For this review, take the finished solid that the model builds, in its own axes (mm). Coordinates: 2 decimals unless noted, no trailing zeros. Loops run counter-clockwise (first coordinate to the right, second up) from the corner with the lowest first, then second, coordinate; pieces in that order, holes last. Notation, with made-up numbers: (-11.75, 77.5) - (44.25, 77.5) arc R17 ccw to (44.25, 93.5) - close; hole circle Ø11 at (36, 69). An arc over 180 degrees is marked (long way). Use one line per item in the form item = value. Start each with the question number.
1. To check wall thickness, follow probe 1 along X at (y, z) = (4, 0); probe 2 along Z at (x, y) = (-102, 1.35); probe 3 along X at (y, z) = (4, 7.5). State the ranges of each line that lie inside material, in increasing order.
2. Add section A-A on z = 20. Give the boundary of the cut face in (x, y), and give its area (3 significant figures).
3. Add section B-B on x = 33. Give the boundary of the cut face in (y, z), and give its area (3 significant figures).
4. Add section C-C on y = 3.65. Give the boundary of the cut face in (x, z) (3 decimals).
```python
from build123d import *

# Parameters (mm, degrees)
SKETCH1_W           = 266.7
SKETCH1_H           = 266.7
SKETCH1_R           = 2.225
SKETCH1_R_2         = 2.5
SKETCH1_W_2         = 225.2
SKETCH1_H_2         = 56.7
BOSS_EXTRUDE1_DEPTH = 5.8
FILLET1_R           = 5.25
CHAMFER1_SIZE       = 1


with BuildPart() as part:
    # Sketch1 → Boss-Extrude1 (new body)
    with BuildSketch(Plane(origin=(0, 0, 0), x_dir=(1, 0, 0), z_dir=(0, 1, 0))):
        Rectangle(SKETCH1_W, SKETCH1_H)
        with Locations(Location((-127.625, 127.625, 0), (0, 0, 270))):
            Circle(SKETCH1_R, mode=Mode.SUBTRACT)
        with Locations(Location((127.625, 127.625, 0), (0, 0, 270))):
            Circle(SKETCH1_R, mode=Mode.SUBTRACT)
        with Locations(Location((127.625, -127.625, 0), (0, 0, 270))):
            Circle(SKETCH1_R, mode=Mode.SUBTRACT)
        with Locations(Location((-127.625, -127.625, 0), (0, 0, 270))):
            Circle(SKETCH1_R, mode=Mode.SUBTRACT)
        with Locations(Location((118.9, 0, 0), (0, 0, 270))):
            Circle(SKETCH1_R_2, mode=Mode.SUBTRACT)
        with Locations(Location((-118.9, 0, 0), (0, 0, 270))):
            Circle(SKETCH1_R_2, mode=Mode.SUBTRACT)
        Rectangle(SKETCH1_W_2, SKETCH1_H_2, mode=Mode.SUBTRACT)
    extrude(amount=BOSS_EXTRUDE1_DEPTH)

    # Fillet1
    fillet1_edges = [part.edges().sort_by_distance(p)[0] for p in [
        (133.35, 2.9, 133.35),
        (-133.35, 2.9, 133.35),
        (-133.35, 2.9, -133.35),
        (133.35, 2.9, -133.35),
    ]]
    fillet(fillet1_edges, radius=FILLET1_R)

    # Chamfer1
    chamfer1_edges = [part.edges().sort_by_distance(p)[0] for p in [
        (112.6, 0, 0),
        (0, 0, -28.35),
        (-112.6, 0, 0),
        (0, 0, 28.35),
        (112.6, 5.8, 0),
        (0, 5.8, -28.35),
        (-112.6, 5.8, 0),
        (0, 5.8, 28.35),
        (-133.35, 0, 0),
        (-133.35, 5.8, 0),
        (133.35, 0, 0),
        (0, 0, 133.35),
        (0, 0, -133.35),
        (-131.812310601, 0, 131.812310601),
        (131.812310601, 0, 131.812310601),
        (131.812310601, 0, -131.812310601),
        (-131.812310601, 0, -131.812310601),
        (0, 5.8, -133.35),
        (133.35, 5.8, 0),
        (0, 5.8, 133.35),
        (-131.812310601, 5.8, 131.812310601),
        (131.812310601, 5.8, 131.812310601),
        (131.812310601, 5.8, -131.812310601),
        (-131.812310601, 5.8, -131.812310601),
    ]]
    chamfer(chamfer1_edges, length=CHAMFER1_SIZE)


solid = part.part
```
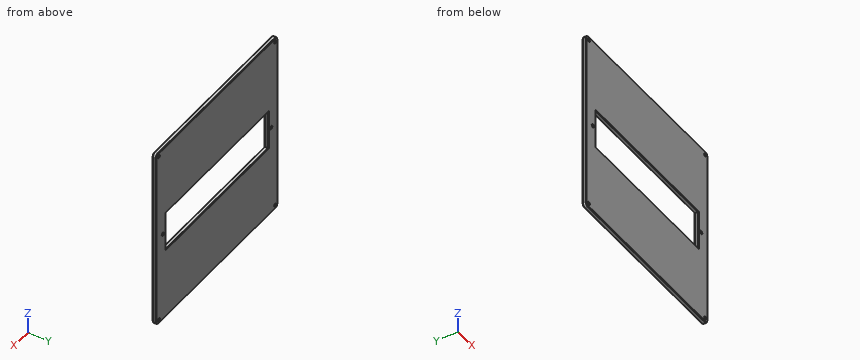
Conclusion:
q1.probe_1 = -133.35 to -121.4, -116.4 to -112.6, 112.6 to 116.4, 121.4 to 133.35
q1.probe_2 = -133.35 to -28.35, 28.35 to 133.35
q1.probe_3 = -133.35 to -112.6, 112.6 to 133.35
q2.outline = (-133.35, 1) - (-132.35, 0) - (-113.6, 0) - (-112.6, 1) - (-112.6, 4.8) - (-113.6, 5.8) - (-132.35, 5.8) - (-133.35, 4.8) - close; (112.6, 1) - (113.6, 0) - (132.35, 0) - (133.35, 1) - (133.35, 4.8) - (132.35, 5.8) - (113.6, 5.8) - (112.6, 4.8) - close
q2.area = 237 mm^2
q3.outline = (0, -132.35) - (1, -133.35) - (4.8, -133.35) - (5.8, -132.35) - (5.8, -29.35) - (4.8, -28.35) - (1, -28.35) - (0, -29.35) - close; (0, 29.35) - (1, 28.35) - (4.8, 28.35) - (5.8, 29.35) - (5.8, 132.35) - (4.8, 133.35) - (1, 133.35) - (0, 132.35) - close
q3.area = 1,210 mm^2
q4.outline = (-133.35, -128.1) arc R5.25 ccw to (-128.1, -133.35) - (128.1, -133.35) arc R5.25 ccw to (133.35, -128.1) - (133.35, 128.1) arc R5.25 ccw to (128.1, 133.35) - (-128.1, 133.35) arc R5.25 ccw to (-133.35, 128.1) - close; hole circle Ø4.45 at (-127.625, -127.625); hole circle Ø4.45 at (-127.625, 127.625); hole circle Ø5 at (-118.9, 0); hole (-112.6, -28.35) - (112.6, -28.35) - (112.6, 28.35) - (-112.6, 28.35) - close; hole circle Ø5 at (118.9, 0); hole circle Ø4.45 at (127.625, -127.625); hole circle Ø4.45 at (127.625, 127.625)
